```python
from build123d import *

# Parameters (mm, degrees)
CROQUIS1_R              = 14.25
CROQUIS1_R_2            = 4.7625
CROQUIS1_R_3            = 19
SALIENTE_EXTRUIR1_DEPTH = 6
REDONDEO1_R             = 25
REDONDEO2_R             = 19.999999878


with BuildPart() as part:
    # Croquis1 → Saliente-Extruir1 (new body)
    with BuildSketch(Plane.XY):
        with BuildLine():
            Line((41.52932014, 201.930330406), (198.68793394, 201.566461221))
            ThreePointArc((198.68793394, 201.566461221), (232.028588704, 169.640855787), (198.25760714, 138.170801026))
            Line((198.25760714, 138.170801026), (65.750390297, 138.369874115))
            Line((65.750390297, 138.369874115), (-93.627365444, -4.467720371))
            ThreePointArc((-93.627365444, -4.467720371), (-138.59478698, -2.355669211), (-136.250697374, 42.600253688))
            Line((-136.250697374, 42.600253688), (41.52932014, 201.930330406))
        make_face()
        with Locations((-115.060486547, 18.956280563)):
            Circle(CROQUIS1_R, mode=Mode.SUBTRACT)
        with Locations((-22.130431971, 105.518425617)):
            Circle(CROQUIS1_R, mode=Mode.SUBTRACT)
        with Locations((200.27932014, 169.856368349)):
            Circle(CROQUIS1_R_2, mode=Mode.SUBTRACT)
        with Locations((70.27932014, 169.856368349)):
            Circle(CROQUIS1_R_2, mode=Mode.SUBTRACT)
        with Locations((-64.936795693, 65.645311557)):
            Circle(CROQUIS1_R_3, mode=Mode.SUBTRACT)
    extrude(amount=SALIENTE_EXTRUIR1_DEPTH)

    # Redondeo1
    redondeo1_edges = [part.edges().sort_by_distance(p)[0] for p in [
        (41.52932014, 201.930330406, 3),
    ]]
    fillet(redondeo1_edges, radius=REDONDEO1_R)

    # Redondeo2
    redondeo2_edges = [part.edges().sort_by_distance(p)[0] for p in [
        (65.750390297, 138.369874115, 3),
    ]]
    fillet(redondeo2_edges, radius=REDONDEO2_R)


solid = part.part
```
The listing builds one solid part. Answer for the finished solid, in the listing's coordinates (mm). Give positions to 0.01 mm unless a question says otherwise; leave off trailing zeros. Write each loop counter-clockwise with the first axis right and the second up, starting at its lowest first coordinate (ties: lowest second). Pieces come first, ordered by that corner, then holes. Notation, with made-up numbers: (-15.5, 75.25) -> (28.5, 75.25) arc R26 ccw to (28.5, 101.25) -> close; hole circle Ø9 at (14, 52). An arc over 180 degrees is marked (long way). Write item = value, one per line. Start each with the question number.
1) Determine the mould class of faces 1 (the face through (-83.92, 66.48, 2.96)), 2 (the face through (43, 119, 6)), 3 (the face through (-138.12, -2.87, 2.96)), 4 (the face through (-15.718, 65.356, 2.958)) for opening direction X: +X half, -X half, draft (parallel to the pull), parting line (faces both ways), or undercut.
2) Straight lines are drawn through the part: line 1 along X through (y, z) = (167.5, 5.4); line 2 along Y through (x, z) = (-104, 1.4); line 3 along Y through (x, z) = (-108, 0.95). For each, find the intervals that lie inside material, in ascending order.
3) The part is cut by section C-C, the plane x = 179. Determine the outline of the cut face in (y, z).
4) The part is cut by section B-B, the plane y = 77.5. Determine the outline of the cut face in (x, z), and give its area (3 significant figures).
5) The part is cut by section A-A, the plane z = 0.95. Count the separate pieces of the cut face and the enclosed holes in it, and give its area (3 significant figures).
6) Each of these flat-tipped pins is pushed along its axis until it touches: pin 1 (1 mm diameter, centred on y = 165.5, z = 5, fed in from -X); pin 2 (2 mm diameter, centred on y = 143, z = 5, fed in from +X). Where does it stop, or does it pass through?
7) The part is cut by section D-D, the plane y = 178.5. Determine the outline of the cut face in (x, z), and give its area (3 significant figures).
Solutions:
q1.face_1 = undercut
q1.face_2 = draft
q1.face_3 = parting line
q1.face_4 = +X half
q2.line_1 = 3.11 to 66.14, 74.42 to 196.14, 204.42 to 231.94
q2.line_2 = -10.8 to 9.97, 27.94 to 71.5
q2.line_3 = -12 to 6.58, 31.33 to 67.92
q3.outline = (138.2, 0) -> (201.61, 0) -> (201.61, 6) -> (138.2, 6) -> close
q4.outline = (-97.31, 0) -> (-79.78, 0) -> (-79.78, 6) -> (-97.31, 6) -> close; (-50.09, 0) -> (-2.17, 0) -> (-2.17, 6) -> (-50.09, 6) -> close
q4.area = 393 mm²
q5.separate_pieces = 1
q5.enclosed_holes = 5
q5.area = 24,300 mm²
q6.pin_1 = 0.32
q6.pin_2 = 218.71
q7.outline = (15.39, 0) -> (230.83, 0) -> (230.83, 6) -> (15.39, 6) -> close
q7.area = 1,290 mm²
